Check sheet for the drawn part. Datum: minimum x, y, z corner. Units: mm. Round coordinates to 2 decimals unless told otherwise and drop trailing zeros. Write each loop counter-clockwise with the first axis right and the second up, starting at its lowest first coordinate (ties: lowest second). Pieces come first, ordered by that corner, then holes. Notation, with made-up numbers: (-23.75, 42.25) - (1.25, 42.25) arc R24 cw to (1.25, 78.25) - close; hole circle Ø9 at (21, 16). An arc over 180 degrees is marked (long way). Answer as a JSON object with one key per item and string values. Group by question number.
Item 1: Gauge pin test, flat ends, axial feed: P1, Ø6, axis at x = 4, y = 30.5, coming from the +Z side; P2, Ø1.5, axis at x = 19.5, z = 52.5, coming from the -Y side; P3, Ø12, axis at x = 28.5, z = 72, coming from the -Y side. Record the tip position at first contact, or that the pin passes through.
Item 2: Sectioned sample at A-A on z = 26.5. Record the boundary of the cut face in (x, y), plus the area to 3 significant figures.
Item 3: Thickness scan on line 1 (Z direction, x = 27, y = 24); line 2 (X direction, y = 13, z = 11); line 3 (Y direction, x = 5.5, z = 51). Record the ranges inside material, lowest first.
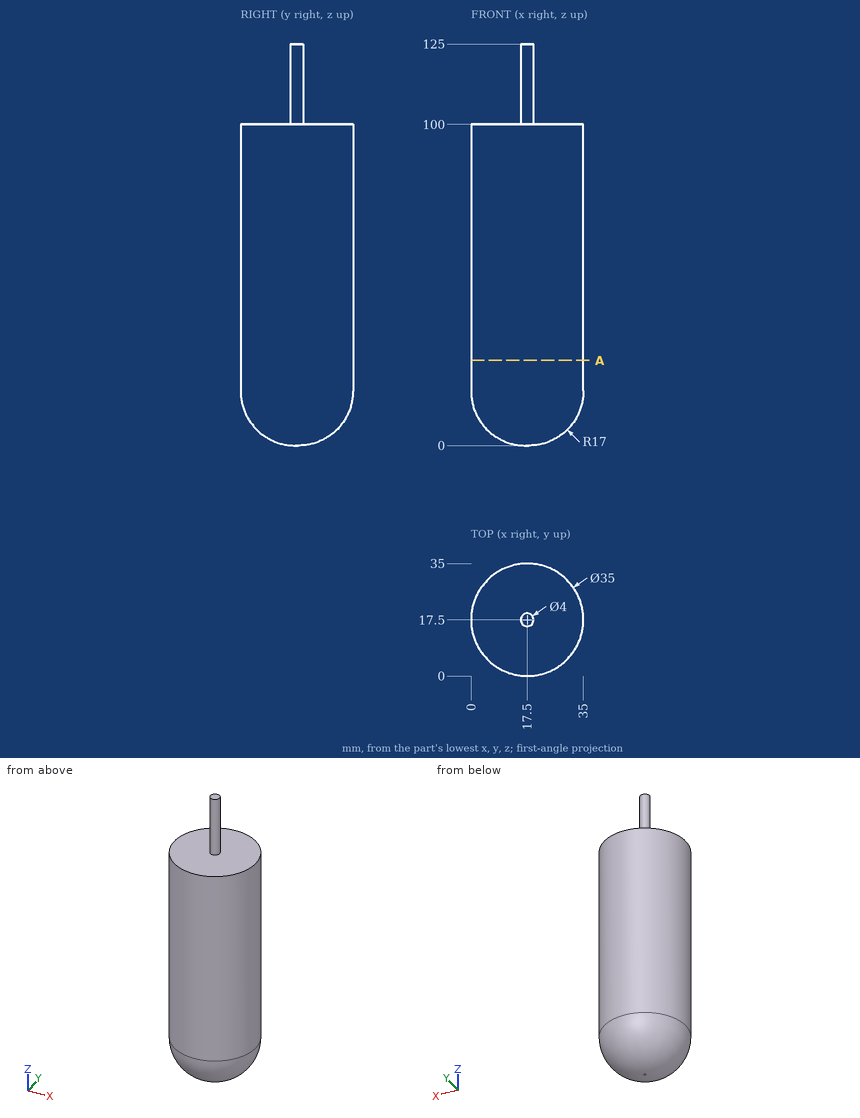
Completed:
{
 "1": {"P1": "z = 100", "P2": "y = 0.04", "P3": "y = 0.73"},
 "2": {"outline": "circle Ø35 at (17.5, 17.5)", "area": "962 mm²"},
 "3": {"line 1": "4.05 to 100", "line 2": "1.72 to 33.28", "line 3": "4.76 to 30.24"}
}
